```python
from build123d import *

# Parameters (mm, degrees)
EXTRUDE_2_DEPTH     = 4
SKETCH_6_R          = 1.6
CUT_EXTRUDE_2_DEPTH = 4
FILLET_START        = -1
FILLET_2_DEPTH      = 6
FILLET_2_2_DEPTH    = 4


with BuildPart() as part:
    # Sketch 1 → Extrude 2 (new body)
    with BuildSketch(Plane(origin=(0, 0, 0), x_dir=(1, 0, 0), z_dir=(0, 1, 0))):
        Polygon((-62.6, 15), (-52.6, 15), (-42.6, 5), (42.6, 5), (52.6, 15), (62.6, 15), (62.6, -15), (-62.6, -15), align=None)
    extrude(amount=EXTRUDE_2_DEPTH)

    # Sketch 6 → Cut-Extrude 2 (cut)
    with BuildSketch(Plane(origin=(0, 4, 0), x_dir=(1, 0, 0), z_dir=(0, 1, 0))):
        with Locations(Location((-53.6, -10, 0), (0, 0, 270))):
            Circle(SKETCH_6_R)
        with Locations(Location((-4, -10, 0), (0, 0, 270))):
            Circle(SKETCH_6_R)
        with Locations(Location((4, -10, 0), (0, 0, 90))):
            Circle(SKETCH_6_R)
        with Locations(Location((53.6, -10, 0), (0, 0, 90))):
            Circle(SKETCH_6_R)
    extrude(amount=-CUT_EXTRUDE_2_DEPTH, mode=Mode.SUBTRACT)

    # Fillet 2: read off the stored shape, not the designer's step
    # Fillet 2 outline → Fillet 2 (cut)
    with BuildSketch(Plane(origin=(0, 0, 0), x_dir=(1, 0, 0), z_dir=(0, 1, 0)).offset(FILLET_START)):
        with BuildLine():
            Line((62.6, -15), (62.6, -12))
            add(Edge.make_bspline(
                [(62.6, -12), (62.6, -15), (59.6, -15)],
                knots=[0, 0, 0, 1, 1, 1], degree=2, weights=[1, 0.707106781, 1]))
            Line((59.6, -15), (62.6, -15))
        make_face()
        with BuildLine():
            add(Edge.make_bspline(
                [(59.6, 15), (62.6, 15), (62.6, 12)],
                knots=[0, 0, 0, 1, 1, 1], degree=2, weights=[1, 0.707106781, 1]))
            Line((62.6, 12), (62.6, 15))
            Line((62.6, 15), (59.6, 15))
        make_face()
        with BuildLine():
            Line((-62.6, -15), (-59.6, -15))
            add(Edge.make_bspline(
                [(-59.6, -15), (-62.6, -15), (-62.6, -12)],
                knots=[0, 0, 0, 1, 1, 1], degree=2, weights=[1, 0.707106781, 1]))
            Line((-62.6, -12), (-62.6, -15))
        make_face()
        with BuildLine():
            add(Edge.make_bspline(
                [(51.721320344, 14.121320344), (52.6, 15), (53.842640687, 15)],
                knots=[0, 0, 0, 1, 1, 1], degree=2, weights=[1, 0.923879533, 1]))
            Line((53.842640687, 15), (52.6, 15))
            Line((52.6, 15), (51.721320344, 14.121320344))
        make_face()
        with BuildLine():
            Line((-62.6, 15), (-62.6, 12))
            add(Edge.make_bspline(
                [(-62.6, 12), (-62.6, 15), (-59.6, 15)],
                knots=[0, 0, 0, 1, 1, 1], degree=2, weights=[1, 0.707106781, 1]))
            Line((-59.6, 15), (-62.6, 15))
        make_face()
        with BuildLine():
            Line((-52.6, 15), (-53.842640687, 15))
            add(Edge.make_bspline(
                [(-53.842640687, 15), (-52.6, 15), (-51.721320344, 14.121320344)],
                knots=[0, 0, 0, 1, 1, 1], degree=2, weights=[1, 0.923879533, 1]))
            Line((-51.721320344, 14.121320344), (-52.6, 15))
        make_face()
    extrude(amount=FILLET_2_DEPTH, mode=Mode.SUBTRACT)

    # Fillet 2 2 outline → Fillet 2 2 (add)
    with BuildSketch(Plane(origin=(0, 0, 0), x_dir=(1, 0, 0), z_dir=(0, 1, 0))):
        with BuildLine():
            Line((42.6, 5), (43.478679656, 5.878679656))
            add(Edge.make_bspline(
                [(41.357359313, 5), (42.6, 5), (43.478679656, 5.878679656)],
                knots=[0, 0, 0, 1, 1, 1], degree=2, weights=[1, 0.923879533, 1]))
            Line((41.357359313, 5), (42.6, 5))
        make_face()
        with BuildLine():
            Line((-42.6, 5), (-41.357359313, 5))
            add(Edge.make_bspline(
                [(-43.478679656, 5.878679656), (-42.6, 5), (-41.357359313, 5)],
                knots=[0, 0, 0, 1, 1, 1], degree=2, weights=[1, 0.923879533, 1]))
            Line((-43.478679656, 5.878679656), (-42.6, 5))
        make_face()
    extrude(amount=FILLET_2_2_DEPTH)


solid = part.part
```
Input: part model. Units: mm. Frame: model coordinates. A direction names the side the tool comes from. Coordinates: 2 decimals unless noted, no trailing zeros. Loops run counter-clockwise (first coordinate to the right, second up) from the corner with the lowest first, then second, coordinate; pieces in that order, holes last. Notation, with made-up numbers: M 6,6.25 L 41,6.25 A25 ccw 41,34.25 Z; hole C -19.75,28.5 d4. An arc over 180 degrees is marked long. Answer in a Markdown table with one row per item.
1. Reachability of faces 4 (the flat face through (62.6, 2, 0)), 5 (the flat face through (-47.7, 2, -10.1)) from +Z, -Z, +X, -X, +Y, -Y: full face, straight path, thin tool, end or side. Return the list, or none.
Response:
| item | result |
|---|---|
| face 4 | +Z, -Z, +X, +Y, -Y |
| face 5 | -Z, +Y, -Y |
2. Material intervals for line 1 (X direction, y = 2.65, z = 10); line 2 (Z direction, x = 19.5, y = 3.3); line 3 (Z direction, x = 5, y = 1.85), sorted ascending.
Response:
| item | result |
|---|---|
| line 1 | x = -62.6 to -55.2, -52 to -5.6, -2.4 to 2.4, 5.6 to 52, 55.2 to 62.6 |
| line 2 | z = -5 to 15 |
| line 3 | z = -5 to 8.75, 11.25 to 15 |
3. Draft query along Z for faces 1 (the flat face through (-1, 4, 3)), 2 (the cylindrical face through (-53.53, 2.03, 8.4)), 3 (the flat face through (-1, 2, -5)). Return one class per face: pulls with the +Z half, pulls with the -Z half, needs draft (parallel to the pull), parting line crosses it, or undercut.
Response:
| item | result |
|---|---|
| face 1 | needs draft |
| face 2 | undercut |
| face 3 | pulls with the -Z half |
4. Section A-A, the plane z = -10. Output: boundary loops of the cut face in (x, y).
Response:
| item | result |
|---|---|
| outline | M -62.6,0 L -47.6,0 L -47.6,4 L -62.6,4 Z; M 47.6,0 L 62.6,0 L 62.6,4 L 47.6,4 Z |
5. First-contact query: pin 1 (4 mm diameter, centred on x = -4, z = 10, fed in from +Y); pin 2 (2 mm diameter, centred on x = 16.5, y = 2.5, fed in from -Z). Flat tips, straight axial feed; report the tip coordinate or a pass-through.
Response:
| item | result |
|---|---|
| pin 1 | stops at y = 4 |
| pin 2 | stops at z = -5 |
6. Section B-B, the plane x = 4. Output: boundary loops of the cut face in (y, z).
Response:
| item | result |
|---|---|
| outline | M 0,-5 L 4,-5 L 4,8.4 L 0,8.4 Z; M 0,11.6 L 4,11.6 L 4,15 L 0,15 Z |
7. Section D-D, the plane x = 23.5. Output: boundary loops of the cut face in (y, z), then the cut area to 3 significant figures.
Response:
| item | result |
|---|---|
| outline | M 0,-5 L 4,-5 L 4,15 L 0,15 Z |
| area | 80.0 mm2 |
8. Section C-C, the plane y = 1. Count the separate pieces of the cut face and the enclosed holes in it, then the cut area to 3 significant figures.
Response:
| item | result |
|---|---|
| separate pieces | 1 |
| enclosed holes | 4 |
| area | 2,760 mm2 |
